```python
from build123d import *

# Parameters (mm, degrees)
SKETCH1_W                     = 44.45
SKETCH1_H                     = 44.45
BOSS_EXTRUDE1_DEPTH           = 8.128
SKETCH2_R                     = 11.05
CUT_EXTRUDE1_DEPTH            = 7
SKETCH3_R                     = 1.905
SKETCH3_R_2                   = 5.715
CUT_EXTRUDE2_DEPTH            = 64.250335967
CBORE_FOR_M3_SHCS1_AT_2_COUNT = 2
CBORE_FOR_M3_SHCS1_AT_2_PITCH = 33.02
CBORE_FOR_M3_SHCS1_AT_3_COUNT = 2
CBORE_FOR_M3_SHCS1_AT_3_PITCH = 46.69733183
CBORE_FOR_M3_SHCS1_AT_4_COUNT = 2
CBORE_FOR_M3_SHCS1_AT_4_PITCH = 33.02
CHAMFER1_SIZE                 = 0.635
CHAMFER2_SIZE                 = 0.635


with BuildPart() as part:
    # Sketch1 → Boss-Extrude1 (new body)
    with BuildSketch(Plane(origin=(0, 0, 0), x_dir=(1, 0, 0), z_dir=(0, 1, 0))):
        with Locations((22.225, 22.225)):
            Rectangle(SKETCH1_W, SKETCH1_H)
    extrude(amount=BOSS_EXTRUDE1_DEPTH)

    # Sketch2 → Cut-Extrude1 (cut)
    with BuildSketch(Plane(origin=(0, 8.128, 0), x_dir=(1, 0, 0), z_dir=(0, 1, 0))):
        with Locations(Location((22.225, 22.225, 0), (0, 0, 270))):
            Circle(SKETCH2_R)
    extrude(amount=-CUT_EXTRUDE1_DEPTH, mode=Mode.SUBTRACT)

    # Sketch3 → Cut-Extrude2 (cut, through all)
    with BuildSketch(Plane(origin=(0, 1.128, 0), x_dir=(1, 0, 0), z_dir=(0, 1, 0))):
        with Locations(Location((22.225, 30.861, 0), (0, 0, 270))):
            Circle(SKETCH3_R)
        with Locations(Location((30.861, 22.225, 0), (0, 0, 270))):
            Circle(SKETCH3_R)
        with Locations(Location((22.225, 13.589, 0), (0, 0, 270))):
            Circle(SKETCH3_R)
        with Locations(Location((13.589, 22.225, 0), (0, 0, 270))):
            Circle(SKETCH3_R)
        with Locations(Location((22.225, 22.225, 0), (0, 0, 270))):
            Circle(SKETCH3_R_2)
    extrude(amount=-CUT_EXTRUDE2_DEPTH, mode=Mode.SUBTRACT)

    # Sketch8 → CBORE for M3 SHCS1 (revolve, cut)
    with BuildSketch(Plane(origin=(5.715, 8.128, -38.735), x_dir=(0, 0, 1), z_dir=(1, 0, 0))):
        Polygon((0, 0), (0, 8.128), (1.7, 8.128), (1.7, 3), (3.25, 3), (3.25, 0.025), (3.275, 0), align=None)
    cbore_for_m3_shcs1 = revolve(axis=Axis((5.715, 14.478, -38.735), (0, -1, 0)), mode=Mode.SUBTRACT)

    # CBORE for M3 SHCS1 at 2: CBORE for M3 SHCS1 ×2
    with Locations(*[(i * CBORE_FOR_M3_SHCS1_AT_2_PITCH, 0, 0) for i in range(1, CBORE_FOR_M3_SHCS1_AT_2_COUNT)]):
        add(cbore_for_m3_shcs1, mode=Mode.SUBTRACT)

    # CBORE for M3 SHCS1 at 3: CBORE for M3 SHCS1 ×2
    with Locations(*[Vector(0.7071067811865477, 0, 0.7071067811865475) * (i * CBORE_FOR_M3_SHCS1_AT_3_PITCH) for i in range(1, CBORE_FOR_M3_SHCS1_AT_3_COUNT)]):
        add(cbore_for_m3_shcs1, mode=Mode.SUBTRACT)

    # CBORE for M3 SHCS1 at 4: CBORE for M3 SHCS1 ×2
    with Locations(*[(0, 0, i * CBORE_FOR_M3_SHCS1_AT_4_PITCH) for i in range(1, CBORE_FOR_M3_SHCS1_AT_4_COUNT)]):
        add(cbore_for_m3_shcs1, mode=Mode.SUBTRACT)

    # Chamfer1
    chamfer1_edges = [part.edges().sort_by_distance(p)[0] for p in [
        (44.45, 8.128, -22.225),
        (22.225, 8.128, -44.45),
        (0, 8.128, -22.225),
        (22.225, 0, -44.45),
        (44.45, 0, -22.225),
        (22.225, 0, 0),
        (0, 0, -22.225),
        (44.45, 4.064, -44.45),
        (44.45, 4.064, 0),
        (22.225, 8.128, 0),
    ]]
    chamfer(chamfer1_edges, length=CHAMFER1_SIZE)

    # Chamfer2
    chamfer2_edges = [part.edges().sort_by_distance(p)[0] for p in [
        (22.225, 8.128, -33.275),
    ]]
    chamfer(chamfer2_edges, length=CHAMFER2_SIZE)


solid = part.part
```
Geometry: final body of the model. Coordinates: model frame, mm. A direction names the side the tool comes from. Round coordinates to 2 decimals unless told otherwise and drop trailing zeros. Write each loop counter-clockwise with the first axis right and the second up, starting at its lowest first coordinate (ties: lowest second). Pieces come first, ordered by that corner, then holes. Notation, with made-up numbers: (-13, -13.75) -> (7, -13.75) arc R18 cw to (7, 8.25) -> close; hole circle Ø7 at (35, -17). An arc over 180 degrees is marked (long way). Return JSON: item names as keys, results as strings.
Q1. Section B-B on z = -21. Give the number of separate pieces and of enclosed holes in the cut face, and give its area (3 significant figures).
From the geometry:
{"separate pieces": "4", "enclosed holes": "0", "area": "187 mm2"}
Q2. Set-up query: faces 5 (the flat face through (32, 8.128, -13)), 6 (the cylindrical face through (5.57, 6.64, -41.98)). Return all of +Z, -Z, +X, -X, +Y, -Y with unobstructed straight access to the full face (end or side cutting, diameter ignored); none if empty.
From the geometry:
{"face 5": "+Z, -Z, +X, -X, +Y", "face 6": "+Y"}
Q3. Ray query, line 1 (Z direction, x = 41.5, y = 5.5); line 2 (Z direction, x = 3, y = 8); line 3 (X direction, y = 2, z = -38.5). Return the intervals inside material, ascending.
From the geometry:
{"line 1": "-44.45 to -40.44, -37.03 to -7.42, -4.01 to 0", "line 2": "-43.94 to -40.52, -36.95 to -7.5, -3.93 to -0.51", "line 3": "0 to 4.03, 7.4 to 37.05, 40.42 to 44.45"}
Q4. Section A-A on y = 6.25. Return the cut outline in (x, z) (3 decimals), and give its area (3 significant figures).
From the geometry:
{"outline": "(0, -44.45) -> (43.815, -44.45) -> (44.45, -43.815) -> (44.45, -0.635) -> (43.815, 0) -> (0, 0) -> close; hole circle Ø6.5 at (5.715, -38.735); hole circle Ø6.5 at (5.715, -5.715); hole circle Ø22.1 at (22.225, -22.225); hole circle Ø6.5 at (38.735, -38.735); hole circle Ø6.5 at (38.735, -5.715)", "area": "1,460 mm2"}
Q5. Mould query, pull axis Z, two halves, no side actions, for faces 1 (the flat face through (44.45, 4, -22)), 2 (the cylindrical face through (5.64, 2.6, -40.433)), 3 (the flat face through (22, 4, 0)), 4 (the flat face through (7.1, 5.128, -40.1)). Classes: +Z half, -Z half, draft (parallel to the pull), parting line (faces both ways), or undercut.
From the geometry:
{"face 1": "draft", "face 2": "undercut", "face 3": "+Z half", "face 4": "undercut"}
Q6. Section D-D on y = 3. Return the cut outline in (x, z) (3 decimals).
From the geometry:
{"outline": "(0, -44.45) -> (43.815, -44.45) -> (44.45, -43.815) -> (44.45, -0.635) -> (43.815, 0) -> (0, 0) -> close; hole circle Ø3.4 at (5.715, -38.735); hole circle Ø3.4 at (5.715, -5.715); hole circle Ø22.1 at (22.225, -22.225); hole circle Ø3.4 at (38.735, -38.735); hole circle Ø3.4 at (38.735, -5.715)"}
Q7. First-contact query: pin 1 Ø18.5 at (x, z) = (22.225, -22.225) entering from +Y; pin 2 Ø3 at (x, z) = (40, -5) entering from +Y. Flat tips, straight axial feed; report the tip coordinate or a pass-through.
From the geometry:
{"pin 1": "y = 1.13", "pin 2": "y = 5.13"}
